Part model, mm, in its own coordinate system. A direction names the side the tool comes from. Give positions to 0.01 mm unless a question says otherwise; leave off trailing zeros. Order: outer loops, then holes, each group sorted by start corner. A loop starts at its lowest first (then second) coordinate and runs counter-clockwise, first axis right, second up. Notation, with made-up numbers: (14.25, 66.5) -> (59.25, 66.5) arc R25 ccw to (59.25, 86.5) -> close; hole circle Ø5 at (47, 84). An arc over 180 degrees is marked (long way). Write item = value, one per line. Start each with the question number.
(1) Saw through at A-A, the plane y = 0. List the corners of the cut face in (x, z).
(2) Probe line 1 along Y through (x, z) = (0, 0.95); line 2 along Y through (x, z) = (0, 7); line 3 along X through (y, z) = (-2.25, 6.25) (3 decimals). List the from-to ranges inside material, lowest first. Write a range as from..to.
(3) Saw through at D-D, the plane z = 0.75. List the corners of the cut face in (x, y), then the cut area to 3 significant figures.
(4) Two-plate mould, pull along Y, no slides. Class faces 1 (the cylindrical face through (9.69, 3.05, 7.26)), 2 (the cylindrical face through (0.54, -2.44, 1.97)), 3 (the flat face through (4.4, -2.1, 8)): pulls with the +Y half, pulls with the -Y half, needs draft (parallel to the pull), parting line crosses it, or undercut.
(5) Flat gauge pins, fed straight in: pin 1 (4 mm diameter, centred on x = 3, z = 4, fed in from -Y); pin 2 (3 mm diameter, centred on y = -1.5, z = 2.5, fed in from +X); pin 3 (1 mm diameter, centred on x = -5, z = 1, fed in from -Y). Where does each tip first touch, or does it go through?
(6) Saw through at C-C, the plane z = 7. List the corners of the cut face in (x, y), then the cut area to 3 significant figures.
(7) Which spindle directions (+Z, -Z, +X, -X, +Y, -Y) get a long thin tool onto all of the face, cutting with end or side? Do faces 4 (the flat face through (-2, -2, 4)), 5 (the flat face through (-2, -2, 0)). Say none if no direction does.
from build123d import *

# Parameters (mm, degrees)
SKETCH1_R           = 10.16
SKETCH1_R_2         = 4.5
BOSS_EXTRUDE1_DEPTH = 8
SKETCH6_R           = 4.5
SKETCH6_R_2         = 2.5
BOSS_EXTRUDE2_DEPTH = 4


with BuildPart() as part:
    # Sketch1 → Boss-Extrude1 (new body)
    with BuildSketch(Plane.XY):
        Circle(SKETCH1_R)
        Circle(SKETCH1_R_2, mode=Mode.SUBTRACT)
    extrude(amount=BOSS_EXTRUDE1_DEPTH)

    # Sketch2 → Cut-Revolve1 (revolve, cut)
    with BuildSketch(Plane(origin=(0, 0, 0), x_dir=(0, 0, -1), z_dir=(1, 0, 0))):
        with BuildLine():
            Line((-6.54, 10.16), (-1.46, 10.16))
            ThreePointArc((-1.46, 10.16), (-4, 7.62), (-6.54, 10.16))
        make_face()
    revolve(axis=Axis((0, 0, 0), (0, 0, 1)), mode=Mode.SUBTRACT)

    # Sketch6 → Boss-Extrude2 (add)
    with BuildSketch(Plane(origin=(0, 0, 0), x_dir=(-1, 0, 0), z_dir=(0, 0, -1))):
        Circle(SKETCH6_R)
        Circle(SKETCH6_R_2, mode=Mode.SUBTRACT)
    extrude(amount=-BOSS_EXTRUDE2_DEPTH)


solid = part.part
Results list:
q1.outline = (-10.16, 0) -> (-2.5, 0) -> (-2.5, 4) -> (-4.5, 4) -> (-4.5, 8) -> (-10.16, 8) -> (-10.16, 6.54) arc R2.54 cw to (-10.16, 1.46) -> close; (2.5, 0) -> (10.16, 0) -> (10.16, 1.46) arc R2.54 cw to (10.16, 6.54) -> (10.16, 8) -> (4.5, 8) -> (4.5, 4) -> (2.5, 4) -> close
q2.line_1 = -10.16..-2.5, 2.5..10.16
q2.line_2 = -10.16..-4.5, 4.5..10.16
q2.line_3 = -8.695..-3.897, 3.897..8.695
q3.outline = circle Ø20.32 at (0, 0); hole circle Ø5 at (0, 0)
q3.area = 305 mm^2
q4.face_1 = parting line crosses it
q4.face_2 = undercut
q4.face_3 = needs draft
q5.pin_1 = -8.14
q5.pin_2 = 10.15
q5.pin_3 = -9.11
q6.outline = circle Ø20.32 at (0, 0); hole circle Ø9 at (0, 0)
q6.area = 261 mm^2
q7.face_4 = +Z
q7.face_5 = -Z, +X, -X, +Y, -Y
